```python
from build123d import *

# Parameters (mm, degrees)
SM_BASE_FLANGE_1_DEPTH = 50
SKETCH_3_R             = 6.5
CUT_EXTRUDE_2_DEPTH    = 101.920760996
SKETCH_5_R             = 11
CUT_EXTRUDE_5_DEPTH    = 101.920760996
SKETCH_6_W             = 4
SKETCH_6_H             = 34
EXTRUDE_2_DEPTH        = 10
CHAMFER_1_SIZE         = 3
CUT_EXTRUDE_6_DEPTH    = 107.230880633
PATTERN_LINEAR_3_COUNT = 2
PATTERN_LINEAR_3_PITCH = 30
FILLET_1_R             = 2
M4X0_7_1_D             = 3.3


# Sheet-metal steps are written as plain solids
with BuildPart() as part:
    # Sketch 1 → 基材-凸緣1 (new body)
    with BuildSketch(Plane(origin=(0, 0, 0), x_dir=(1, 0, 0), z_dir=(0, 1, 0))):
        with BuildLine():
            Line((31, 0), (4.7366, 0))
            ThreePointArc((4.7366, 0), (1.38731802, 1.38731802), (0, 4.7366))
            Line((0, 4.7366), (0, 82))
            Line((0, 82), (4, 82))
            Line((4, 82), (4, 4.7366))
            ThreePointArc((4, 4.7366), (4.215745145, 4.215745145), (4.7366, 4))
            Line((4.7366, 4), (31, 4))
            Line((31, 4), (31, 0))
        make_face()
    extrude(amount=SM_BASE_FLANGE_1_DEPTH)

    # 草圖3 → 除料-伸長2 (cut, through all)
    with BuildSketch(Plane.ZY):
        with Locations((-22.7366, 25)):
            Circle(SKETCH_3_R)
    extrude(amount=-CUT_EXTRUDE_2_DEPTH, mode=Mode.SUBTRACT)

    # 草圖5 → 除料-伸長5 (cut, through all)
    with BuildSketch(Plane.ZY):
        with Locations((-64.94145754, 20)):
            Circle(SKETCH_5_R)
    extrude(amount=-CUT_EXTRUDE_5_DEPTH, mode=Mode.SUBTRACT)

    # 草圖6 → 填料-伸長2 (add)
    with BuildSketch(Plane(origin=(0, 50, 0), x_dir=(1, 0, 0), z_dir=(0, 1, 0))):
        with Locations((2, 65)):
            Rectangle(SKETCH_6_W, SKETCH_6_H)
    extrude(amount=EXTRUDE_2_DEPTH)

    # 導角1
    chamfer_1_edges = [part.edges().sort_by_distance(p)[0] for p in [
        (31, 50, -2),
        (2, 60, -48),
        (2, 60, -82),
        (31, 0, -2),
        (2, 0, -82),
    ]]
    chamfer(chamfer_1_edges, length=CHAMFER_1_SIZE)

    # 草圖8 → 除料-伸長6 (cut, through all)
    with BuildSketch(Plane.XY):
        with BuildLine():
            Line((19.6, 42.6), (24.6, 42.6))
            ThreePointArc((24.6, 42.6), (27.2, 40), (24.6, 37.4))
            Line((24.6, 37.4), (19.6, 37.4))
            ThreePointArc((19.6, 37.4), (17, 40), (19.6, 42.6))
        make_face()
    cut_extrude_6 = extrude(amount=-CUT_EXTRUDE_6_DEPTH, mode=Mode.SUBTRACT)

    # 直線複製排列3: 除料-伸長6 ×2
    with Locations(*[(0, -i * PATTERN_LINEAR_3_PITCH, 0) for i in range(1, PATTERN_LINEAR_3_COUNT)]):
        add(cut_extrude_6, mode=Mode.SUBTRACT)

    # 圓角1
    fillet_1_edges = [part.edges().sort_by_distance(p)[0] for p in [
        (2, 50, -48),
    ]]
    fillet(fillet_1_edges, radius=FILLET_1_R)

    # M4x0.7 螺紋孔1 (through all)
    with Locations(Plane.ZY):
        with Locations((-59.94145754, 5), (-69.94145754, 5), (-69.94145754, 54.5), (-59.94145754, 54.5)):
            Hole(M4X0_7_1_D / 2)


solid = part.part
```
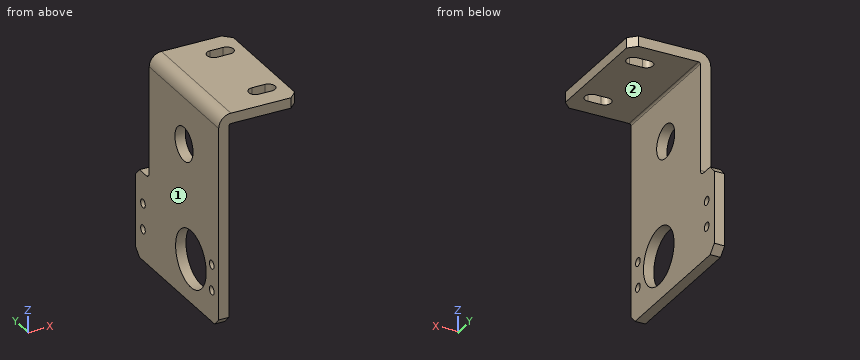
Can you work these out from the model? Positions are in its coordinate system, mm. Face numbers are marked on the shaded views. A direction names the side the tool comes from. Coordinates: 2 decimals unless noted, no trailing zeros. Order: outer loops, then holes, each group sorted by start corner. A loop starts at its lowest first (then second) coordinate and runs counter-clockwise, first axis right, second up. Notation, with made-up numbers: (-35.75, 49.5) - (-7.75, 49.5) arc R12 ccw to (-7.75, 69.5) - close; hole circle Ø9 at (79.5, 77). An arc over 180 degrees is marked (long way). Answer in a Markdown table with one row per item.
1. Suppose I cut it at B-B (y = 27). Please give me the cut outline in (x, z).
Reply:
| item | result |
|---|---|
| outline | (0, -82) - (4, -82) - (4, -73.43) - (0, -73.43) - close; (0, -56.46) - (4, -56.46) - (4, -28.92) - (0, -28.92) - close; (0, -16.55) - (4, -16.55) - (4, -4.74) arc R0.74 cw to (4.74, -4) - (31, -4) - (31, 0) - (4.74, 0) arc R4.74 ccw to (0, -4.74) - close |
2. For pin 1 (4.5 mm diameter, centred on x = 22.5, z = -1, fed in from +Y); pin 2 (1.5 mm diameter, centred on y = 8, z = -41.5, fed in from +X); pin 3 (3 mm diameter, centred on x = 21.5, y = 33, fed in from -Z), each with a flat end and sliding along its axis, tell me the tip position at first contact or that it passes through.
Reply:
| item | result |
|---|---|
| pin 1 | stops at y = 50 |
| pin 2 | stops at x = 4 |
| pin 3 | stops at z = -4 |
3. If I drill on line 1 along Z through (x, y) = (3.5, 21.5); line 2 along Z through (x, y) = (1, 54); line 3 along Z through (x, y) = (11, 15), over which ranges is the centre line in solid material (lowest first)?
Reply:
| item | result |
|---|---|
| line 1 | z = -82 to -75.84, -54.04 to -28.21, -17.26 to -0.16 |
| line 2 | z = -82 to -71.51, -68.37 to -61.51, -58.37 to -48 |
| line 3 | z = -4 to 0 |
4. For the marked faces 1 and 2, which set-ups out of +Z, -Z, +X, -X, +Y, -Y let a thin tool reach every point of the face, with its end or its side?
Reply:
| item | result |
|---|---|
| face 1 | +Z, -Z, -X, +Y, -Y |
| face 2 | -Z, +X, +Y, -Y |
5. Suppose I cut it at D-D (x = 18.5). Please give me the cut outline in (y, z), and give its area (3 significant figures).
Reply:
| item | result |
|---|---|
| outline | (0, -4) - (7.64, -4) - (7.64, 0) - (0, 0) - close; (12.36, -4) - (37.64, -4) - (37.64, 0) - (12.36, 0) - close; (42.36, -4) - (50, -4) - (50, 0) - (42.36, 0) - close |
| area | 162 mm^2 |
6. Suppose I cut it at C-C (z = -25.5). Please give me the cut outline in (x, y), and give its area (3 significant figures).
Reply:
| item | result |
|---|---|
| outline | (0, 0) - (4, 0) - (4, 19.12) - (0, 19.12) - close; (0, 30.88) - (4, 30.88) - (4, 50) - (0, 50) - close |
| area | 153 mm^2 |
7. Suppose I cut it at A-A (y = 40). Please give me the cut outline in (x, z).
Reply:
| item | result |
|---|---|
| outline | (0, -82) - (4, -82) - (4, -4.74) arc R0.74 cw to (4.74, -4) - (17, -4) - (17, 0) - (4.74, 0) arc R4.74 ccw to (0, -4.74) - close; (27.2, -4) - (31, -4) - (31, 0) - (27.2, 0) - close |
